Autodesk Inventor part; units mm, degrees
ref_plane "YZ Plane" through (0, 0, 0) normal (1, 0, 0) x (0, 1, 0)
ref_plane "XZ Plane" through (0, 0, 0) normal (0, 1, 0) x (-1, 0, 0)
ref_plane "XY Plane" through (0, 0, 0) normal (0, 0, 1) x (1, 0, 0)
sketch "스케치18" plane through (0, 0, 0) normal (0, 0, 1) x (1, 0, 0)
  line L0 (55, 0) -> (55, 20)
  line L1 (55, 20) -> (89.63, 20)
  line L2 (89.63, 20) -> (89.63, 41.5)
  line L3 (89.63, 41.5) -> (-89.4, 41.5)
  line L4 (-89.4, 41.5) -> (-89.4, 20)
  line L5 (-89.4, 20) -> (-55, 20)
  line L6 (-55, 20) -> (-55, -55)
  line L7 (55, 0) -> (55, -55)
  line L8 (-55, -55) -> (-55, -99.24)
  line L9 (-55, -99.24) -> (-40.255, -143.4879)
  line L10 (-40.255, -143.4879) -> (40.245, -143.4879)
  line L11 (55, -55) -> (55, -99.24)
  line L12 (55, -99.24) -> (40.245, -143.4879)
  point P0 (0, 0)
  dimension "d111" = 179.03
  dimension "d112" = 184.9879
  dimension "d113" = 34.4
extrude "돌출13" add sketch "스케치18" along normal blind 10
shell "쉘4" thickness 2 removed faces 1 at (-18.3333, -11.6667, 10)
sketch "스케치23" plane through (87.63, 22, 2) normal (-1, 0, 0) x (0, 0, 1)
  line L0 (0, 0) -> (8, 0)
  line L1 (0, 0) -> (0, 17.5)
  line L2 (8, 0) -> (0, 0)
  line L3 (0, 0) -> (0, 17.5)
  line L4 (0, 17.5) -> (8, 17.5)
  line L5 (8, 17.5) -> (8, 0)
  point P0 (-2, -22)
extrude "돌출16" cut sketch "스케치23" along normal mid plane 600
fillet "모깎기6" radius 4 8 edges at (0.115, 41.5, 0) (72.315, 20, 0) (-72.2, 20, 0) (-55, -39.62, 0) (55, -39.62, 0) (47.6225, -121.3639, 0) (-0.005, -143.4879, 0) (-47.6275, -121.3639, 0)
sketch "스케치24" plane through (0, 0, 0) normal (0, 0, -1) x (-1, 0, 0)
  line L0 (0, -98.5907) -> (-13.5, -98.5907)
  line L1 (0, -98.5907) -> (13.5, -98.5907)
  line L2 (-13.5, -98.5907) -> (-13.5, -128.5907)
  line L3 (-13.5, -128.5907) -> (0, -128.5907)
  line L4 (0, -128.5907) -> (13.5, -128.5907)
  line L5 (13.5, -128.5907) -> (13.5, -98.5907)
  line L6 (0, -98.5907) -> (6, -98.5907)
  line L7 (6, -98.5907) -> (6, -102.5907)
  line L8 (6, -102.5907) -> (-6, -102.5907)
  line L9 (-6, -102.5907) -> (-6, -98.5907)
  point P0 (0, 0)
  dimension "d136" = 6
  dimension "d137" = 4
  dimension "d138" = 12
extrude "돌출17" cut sketch "스케치24" against normal blind 1
sketch "스케치25" plane through (0, 0, 1) normal (0, 0, -1) x (-1, 0, 0)
  line L0 (-13.5, -98.5907) -> (13.5, -98.5907)
  line L1 (0, -98.5907) -> (6, -98.5907)
  line L2 (6, -98.5907) -> (6, -102.5907)
  line L3 (6, -102.5907) -> (-6, -102.5907)
  line L4 (-6, -102.5907) -> (-6, -98.5907)
  line L5 (-6, -98.5907) -> (0, -98.5907)
  point P0 (0, 0)
  dimension "d139" = 6
  dimension "d140" = 4
  dimension "d141" = 12
extrude "돌출18" cut sketch "스케치25" against normal blind 2
sketch "스케치26" plane through (0, 0, 0) normal (0, 0, -1) x (-1, 0, 0)
  point P0 (0, 0)
properties part number "8.7_수정본"
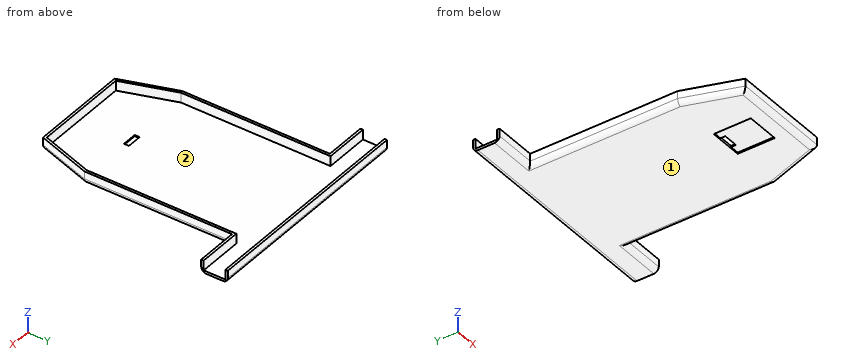
Part model, mm, in its own coordinate system. Face numbers are marked on the shaded views. Give positions to 0.01 mm unless a question says otherwise; leave off trailing zeros. Loops run counter-clockwise (first coordinate to the right, second up) from the corner with the lowest first, then second, coordinate; pieces in that order, holes last.
(1) Drill centre lines: line 1 along X through (y, z) = (-59.5, 9.25); line 2 along Y through (x, z) = (61, 7.25); line 3 along Y through (x, z) = (-26, 4.75). Where is each one in solid material? Low to high.
Return value:
line 1: x = -55 to -53, 53 to 55
line 2: y = 20 to 22, 39.5 to 41.5
line 3: y = -143.49 to -141.49, 39.5 to 41.5
(2) Pull direction X, two halves, no side cores. Call the marked faces 1 and 2: pulls with the +X half, pulls with the -X half, needs draft (parallel to the pull), parting line crosses it, or undercut.
Return value:
face 1: needs draft
face 2: undercut
(3) Band-saw the part on A-A (z = 6). Write the cut outline in (x, y) (3 decimals), and give its area (3 significant figures).
Return value:
outline: (-89.4, 20) - (-55, 20) - (-55, -99.24) - (-40.255, -143.488) - (40.245, -143.488) - (55, -99.24) - (55, 20) - (89.63, 20) - (89.63, 22) - (53, 22) - (53, -98.915) - (38.804, -141.488) - (-38.813, -141.488) - (-53, -98.916) - (-53, 22) - (-89.4, 22) - close; (-89.4, 39.5) - (89.63, 39.5) - (89.63, 41.5) - (-89.4, 41.5) - close
area: 1,320 mm2
(4) Band-saw the part on C-C (y = -26.5). Write the cut outline in (x, z).
Return value:
outline: (-55, 4) arc R4 ccw to (-51, 0) - (51, 0) arc R4 ccw to (55, 4) - (55, 10) - (53, 10) - (53, 2) - (-53, 2) - (-53, 10) - (-55, 10) - close
(5) Pin check, flat tips, straight feed: pin 1 (3 mm diameter, centred on y = -79, z = 8, fed in from -X); pin 2 (6 mm diameter, centred on y = -117, z = 5.5, fed in from +X); pin 3 (0.5 mm diameter, centred on y = -99.5, z = 1.5, fed in from -X). Stop position of each tip, or through.
Return value:
pin 1: stops at x = -55
pin 2: stops at x = 50.08
pin 3: stops at x = -54.2
(6) Band-saw the part on B-B (x = -16.5). Write the cut outline in (y, z), and give its area (3 significant figures).
Return value:
outline: (-143.49, 4) arc R4 ccw to (-139.49, 0) - (37.5, 0) arc R4 ccw to (41.5, 4) - (41.5, 10) - (39.5, 10) - (39.5, 2) - (-141.49, 2) - (-141.49, 10) - (-143.49, 10) - close
area: 395 mm2
